The model under review builds one solid part; all positions refer to its coordinate system, in mm. A direction names the side the tool comes from. Give positions to 0.01 mm unless a question says otherwise; leave off trailing zeros. Order: outer loops, then holes, each group sorted by start corner. A loop starts at its lowest first (then second) coordinate and runs counter-clockwise, first axis right, second up. Notation, with made-up numbers: (-9.75, 25) - (40.25, 25) arc R16 ccw to (40.25, 40) - close; hole circle Ø10 at (-5.75, 44). An arc over 180 degrees is marked (long way). Use CSV: the item, a comma, the result in double quotes.
```python
from build123d import *

# Parameters (mm, degrees)
F0_R     = 2.5
F1_DEPTH = 3


# Not quite as in the source:
# - ends of sketch curves that miss each other by under 0.0002 mm in the source are joined


with BuildPart() as f1:
    # F0 (on Top) → F1 (new body)
    with BuildSketch(Plane.XY):
        Polygon((-34.5, 32), (-47, 32), (-47, 22.4999984801), (-44, 22.4999984801), (-44, 7.4999984801), (-49.5, 7.4999984801), (-49.5, -7.5000015199), (-44, -7.5000015199), (-44, -22.5000015199), (-49.5, -22.5000015199), (-49.5, -32.0000015199), (-34.5, -32), (-34.5, -35), (-24.5, -35), (-24.5, -32), (-14.5, -32), (-14.5, -35), (-4.5, -35), (-4.5, -32), (5.5, -32), (5.5, -35), (15.5, -35), (15.5, -32), (25.5, -32), (25.5, -35), (35.5, -35), (35.5, -32), (40.5, -32), (45.5, -32), (45.5, -35), (55.5, -35), (55.5, -32), (65.5, -32), (65.5, -35), (75.5, -35), (75.5, -32), (85.5, -32), (85.5, -35), (95.5, -35), (95.5, -32), (105.5, -32), (105.5, -35), (115.5, -35), (115.5, -32), (130.5, -32), (130.5, -22.5000015199), (125, -22.5000015199), (125, -7.5000015199), (130.5, -7.5000015199), (130.5, 7.4999984801), (125, 7.4999984801), (125, 22.4999984801), (128, 22.4999984801), (128, 31.9999984801), (115.5, 32), (115.5, 35), (105.5, 35), (105.5, 32), (95.5, 32), (95.5, 35), (85.5, 35), (85.5, 32), (75.5, 32), (75.5, 35), (65.5, 35), (65.5, 32), (55.5, 32), (55.5, 35), (45.5, 35), (45.5, 32), (40.5, 32), (35.5, 32), (35.5, 35), (25.5, 35), (25.5, 32), (15.5, 32), (15.5, 35), (5.5, 35), (5.5, 32), (-4.5, 32), (-4.5, 35), (-14.5, 35), (-14.5, 32), (-24.5, 32), (-24.5, 35), (-34.5, 35), align=None)
        with Locations((-17, -12.5)):
            Circle(F0_R, mode=Mode.SUBTRACT)
        with Locations((55.5, -12.5)):
            Circle(F0_R, mode=Mode.SUBTRACT)
        with Locations((-17, 12.5)):
            Circle(F0_R, mode=Mode.SUBTRACT)
        with Locations((58, 12.5)):
            Circle(F0_R, mode=Mode.SUBTRACT)
    extrude(amount=F1_DEPTH)


solid = f1.part
```
Item 1: Wall thickness on L1, parallel to Y at x = -17, z = 1.15; L2, parallel to X at y = 13, z = 2.4; L3, parallel to Y at x = 80, z = 0.85: over which ranges is each line inside the solid? List them lowest first.
Results list:
L1,"y = -32 to -15, -10 to 10, 15 to 32"
L2,"x = -44 to -19.45, -14.55 to 55.55, 60.45 to 125"
L3,"y = -32 to 32"
Item 2: Clearance check with flat-ended pins moving along their axes: pin 1 (0.9 mm diameter, centred on y = 12, z = 1, fed in from +X); pin 2 (1.5 mm diameter, centred on y = 33.5, z = 2, fed in from +X); pin 3 (0.9 mm diameter, centred on y = -33, z = 2, fed in from -X). State where each tip first meets the part, or that it passes through.
Results list:
pin 1,"stops at x = 125"
pin 2,"stops at x = 115.5"
pin 3,"stops at x = -34.5"
Item 3: Tool access review of faces 1 (the face through (1, 32, 1)), 2 (the face through (-47, 7.5, 1)), 3 (the face through (40, -32, 1)): name each direction out of +Z, -Z, +X, -X, +Y, -Y from which nothing blocks a thin tool from reaching the whole face with its end or side.
Results list:
face 1,"+Z, -Z, +Y"
face 2,"+Z, -Z, -X"
face 3,"+Z, -Z, -Y"
Item 4: Mouldability with a two-part tool opening along X and no side actions: class faces 4 (the face through (-34.5, -33, 1)), 5 (the face through (10, -35, 1)), 6 (the face through (125, 15, 1)), 7 (the face through (15.5, -34, 1)) as pulls with the +X half, pulls with the -X half, needs draft (parallel to the pull), parting line crosses it, or undercut.
Results list:
face 4,"pulls with the -X half"
face 5,"needs draft"
face 6,"pulls with the +X half"
face 7,"undercut"
Item 5: Take a section at C-C, the plane z = 1.65. State how many separate pieces and enclosed holes the cut face has, and give its area (3 significant figures).
Results list:
separate pieces,"1"
enclosed holes,"4"
area,"11,500 mm2"
Item 6: Take a section at D-D, the plane x = 42. Give the boundary of the cut face in (y, z).
Results list:
outline,"(-32, 0) - (32, 0) - (32, 3) - (-32, 3) - close"
Item 7: Take a section at B-B, the plane x = -17. Give the boundary of the cut face in (y, z).
Results list:
outline,"(-32, 0) - (-15, 0) - (-15, 3) - (-32, 3) - close; (-10, 0) - (10, 0) - (10, 3) - (-10, 3) - close; (15, 0) - (32, 0) - (32, 3) - (15, 3) - close"
Item 8: Take a section at A-A, the plane y = -12.5. Give the boundary of the cut face in (x, z).
Results list:
outline,"(-44, 0) - (-19.5, 0) - (-19.5, 3) - (-44, 3) - close; (-14.5, 0) - (53, 0) - (53, 3) - (-14.5, 3) - close; (58, 0) - (125, 0) - (125, 3) - (58, 3) - close"
